CAD build for the part. Positions are in the model's coordinates, mm. Face numbers are marked on the shaded views. A direction names the side the tool comes from. Round coordinates to 2 decimals unless told otherwise and drop trailing zeros. Loops run counter-clockwise (first coordinate to the right, second up) from the corner with the lowest first, then second, coordinate; pieces in that order, holes last.
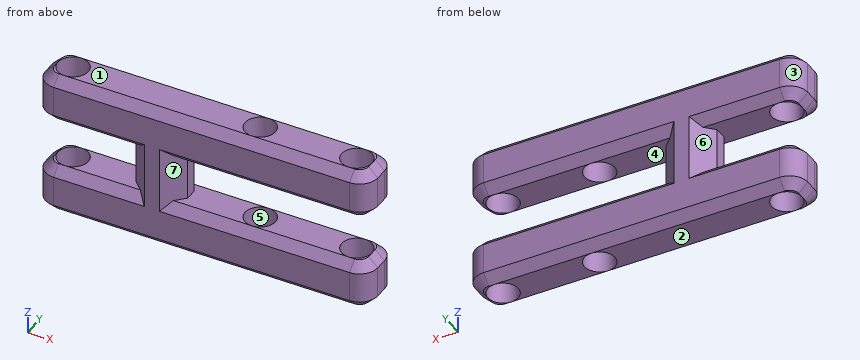
Autodesk Inventor part; units mm, degrees
ref_plane "YZ Plane" through (0, 0, 0) normal (1, 0, 0) x (0, 1, 0)
ref_plane "XZ Plane" through (0, 0, 0) normal (0, 1, 0) x (-1, 0, 0)
ref_plane "XY Plane" through (0, 0, 0) normal (0, 0, 1) x (1, 0, 0)
sketch "Sketch1" plane through (0, 0, 0) normal (0, 0, 1) x (1, 0, 0)
  line L0 (20, 36) -> (-35, 36)
  line L1 (-35, 36) -> (-35, 28)
  line L2 (-35, 28) -> (20, 28)
  line L3 (20, 28) -> (20, 36)
  circle A0 centre (16, 32) radius 2.5
  circle A1 centre (-31, 32) radius 2.5
  arc A2 (-2.5, 32) -> (2.5, 32) centre (0, 32) ccw
  line L4 (-2.5, 32) -> (-2.5, -32)
  line L5 (2.5, -32) -> (2.5, 32)
  arc A3 (2.5, -32) -> (-2.5, -32) centre (0, -32) ccw
  arc A4 (0, 34.5) -> (-2.5, 32) centre (0, 32) ccw
  arc A5 (2.5, 32) -> (0, 34.5) centre (0, 32) ccw
  point P0 (0, 0)
  point P1 (-2.5, 28)
  point P2 (2.5, 28)
  dimension "d0" = 8
  dimension "d2" = 55
  dimension "d4" = 4
  dimension "d5" = 4
  dimension "d7" = 4
  dimension "d11" = 5
extrude "Extrusion1" add sketch "Sketch1" along normal blind 8 contours L3 L2 L5 A5 A4 L4 L1 L0 | L2 L4 A2 L5
fillet "Fillet1" radius 3 4 edges at (-35, 36, 4) (-35, 28, 4) (20, 28, 4) (20, 36, 4)
sketch "Sketch2" plane through (0, 0, 0) normal (0, 0, -1) x (-1, 0, 0)
  arc A0 (-17, 36) -> (-20, 33) centre (-17, 33) ccw
  line L0 (-20, 31) -> (-20, 33)
  arc A1 (-20, 31) -> (-17, 28) centre (-17, 31) ccw
  line L1 (32, 28) -> (-17, 28)
  arc A2 (32, 28) -> (35, 31) centre (32, 31) ccw
  line L2 (35, 33) -> (35, 31)
  arc A3 (35, 33) -> (32, 36) centre (32, 33) ccw
  line L3 (-17, 36) -> (32, 36)
  line L4 (20, 36) -> (32, 36)
  line L5 (32, 28) -> (20, 28)
  line L6 (20, 28) -> (20, 36)
  line L7 (32, 28) -> (-17, 28)
  line L8 (11.5, 36) -> (19.5, 36)
  line L9 (19.5, 36) -> (19.5, 28)
  line L10 (19.5, 28) -> (11.5, 28)
  line L11 (11.5, 28) -> (11.5, 36)
  point P0 (0, 0)
  dimension "d12" = 15
  dimension "d21" = 8
extrude "Extrusion2" add sketch "Sketch2" along normal blind 8 contours L3 L9 L1 L11 | L3 L6 L1 L9
sketch "Sketch3" plane through (0, 0, -8) normal (0, 0, -1) x (-1, 0, 0)
  line L0 (-17, 36) -> (11.5, 36)
  arc A0 (-17, 36) -> (-20, 33) centre (-17, 33) ccw
  line L1 (-20, 31) -> (-20, 33)
  arc A1 (-20, 31) -> (-17, 28) centre (-17, 31) ccw
  line L2 (32, 28) -> (19.5, 28)
  circle A2 centre (0, 32) radius 2.5
  circle A3 centre (-16, 32) radius 2.5
  line L3 (20, 36) -> (11.5, 36)
  line L4 (19.5, 36) -> (19.5, 28)
  arc A4 (32, 28) -> (35, 31) centre (32, 31) ccw
  line L5 (35, 33) -> (35, 31)
  arc A5 (35, 33) -> (32, 36) centre (32, 33) ccw
  line L6 (19.5, 36) -> (32, 36)
  line L7 (11.5, 28) -> (11.5, 36)
  line L8 (11.5, 28) -> (-17, 28)
  circle A6 centre (31, 32) radius 2.5
  line L9 (11.5, 28) -> (20, 28)
  line L10 (20, 28) -> (20, 36)
  line L11 (11.5, 36) -> (11.5, 28)
  point P0 (0, 0)
  point P1 (-17, 36)
extrude "Extrusion3" add sketch "Sketch3" along normal blind 8
chamfer "Chamfer1" distance 3 angle 45 4 edges at (-11.5, 36, -4) (-20, 36, -4) (-20, 28, -4) (-11.5, 28, -4)
chamfer "Chamfer2" distance 1.5 angle 45 44 edges at (-13, 36, 0) (2.75, 36, 0) (19.1213, 35.1213, 0) (20, 32, 0) (19.1213, 28.8787, 0) (-18.5, 28, 0) (2.75, 28, 0) (-13, 28, 0) (-18.5, 36, 0) (-26, 36, 0) (-34.1213, 35.1213, 0) (-35, 32, 0) (-34.1213, 28.8787, 0) (-26, 28, 0) (-18.5, 36, -8) (-26, 36, -8) (-13, 36, -8) (-34.1213, 35.1213, -8) (-35, 32, -8) (-34.1213, 28.8787, -8) (-18.5, 28, -8) (-26, 28, -8) (-13, 28, -8) (2.75, 36, -8) (19.1213, 35.1213, -8) (20, 32, -8) (19.1213, 28.8787, -8) (2.75, 28, -8) (-7.5, 36, -16) (19.1213, 35.1213, -16) (20, 32, -16) (19.1213, 28.8787, -16) (-7.5, 28, -16) (-34.1213, 28.8787, -16) (-35, 32, -16) (-34.1213, 35.1213, -16) (-7.5, 36, 8) (-34.1213, 35.1213, 8) (-35, 32, 8) (-34.1213, 28.8787, 8) (-7.5, 28, 8) (19.1213, 28.8787, 8) (20, 32, 8) (19.1213, 35.1213, 8)
properties part number "cross-beam"
Item 1: 3-axis set-ups, long thin cutter, end or side, ignore diameter. For the marked faces 5, 6 and 7: which of +Z, -Z, +X, -X, +Y, -Y reach the whole face in a straight line?
Answers follow:
face 5: +Z, -Z
face 6: -X, +Y
face 7: +X, -Y
Item 2: Cut at C-C, the plane z = 4.5. Give the cut face in (x, y), plus the area to 3 significant figures.
Answers follow:
outline: (-35, 31) arc R3 ccw to (-32, 28) - (17, 28) arc R3 ccw to (20, 31) - (20, 33) arc R3 ccw to (17, 36) - (-32, 36) arc R3 ccw to (-35, 33) - close; hole circle Ø5 at (-31, 32); hole circle Ø5 at (0, 32); hole circle Ø5 at (16, 32)
area: 373 mm2
Item 3: Flat gauge pins, fed straight in: P1, Ø1, axis at y = 32, z = -3.5, coming from the -X side; P2, Ø3, axis at x = -31, y = 32, coming from the +Z side; P3, Ø0.6, axis at y = 32, z = -4, coming from the +X side; P4, Ø3, axis at y = 34.5, z = -7.5, coming from the -X side. Where does each tip first touch, or does it go through?
Answers follow:
P1: stops at x = -20
P2: passes through
P3: stops at x = -11.5
P4: stops at x = -34.2
Item 4: Cut at D-D, the plane z = -5.5. Give the cut face in (x, y).
Answers follow:
outline: (-20, 31) - (-17, 28) - (-14.5, 28) - (-11.5, 31) - (-11.5, 33) - (-14.5, 36) - (-17, 36) - (-20, 33) - close
Item 5: Probe line 1 (Z direction, x = -10, y = 30); line 2 (Y direction, x = 0, z = 3); line 3 (X direction, y = 34, z = 1.5). List the from-to ranges inside material, lowest first.
Answers follow:
line 1: z = -16 to -8, 0 to 8
line 2: y = 28 to 29.5, 34.5 to 36
line 3: x = -34.83 to -32.5, -29.5 to -1.5, 1.5 to 14.5, 17.5 to 19.83
Item 6: Cut at B-B, the plane x = -25. Give the cut face in (y, z), plus the area to 3 significant figures.
Answers follow:
outline: (28, -14.5) - (29.5, -16) - (34.5, -16) - (36, -14.5) - (36, -9.5) - (34.5, -8) - (29.5, -8) - (28, -9.5) - close; (28, 1.5) - (29.5, 0) - (34.5, 0) - (36, 1.5) - (36, 6.5) - (34.5, 8) - (29.5, 8) - (28, 6.5) - close
area: 119 mm2
Item 7: Two-plate mould, pull along Z, no slides. Class the marked faces 1, 2, 3 and 4: released by +Z, released by -Z, zero draft, split by the parting line, or undercut.
Answers follow:
face 1: released by +Z
face 2: released by -Z
face 3: zero draft
face 4: undercut
Item 8: Cut at A-A, the plane x = 14.5. Give the cut face in (y, z), plus the area to 3 significant figures.
Answers follow:
outline: (28, -14.5) - (29.5, -16) - (30, -16) - (30, -8) - (29.5, -8) - (28, -9.5) - close; (28, 1.5) - (29.5, 0) - (30, 0) - (30, 8) - (29.5, 8) - (28, 6.5) - close; (34, -16) - (34.5, -16) - (36, -14.5) - (36, -9.5) - (34.5, -8) - (34, -8) - close; (34, 0) - (34.5, 0) - (36, 1.5) - (36, 6.5) - (34.5, 8) - (34, 8) - close
area: 55.0 mm2
